Autodesk Inventor part; units mm, degrees
ref_plane "YZ Plane" through (0, 0, 0) normal (1, 0, 0) x (0, 1, 0)
ref_plane "XZ Plane" through (0, 0, 0) normal (0, 1, 0) x (-1, 0, 0)
ref_plane "XY Plane" through (0, 0, 0) normal (0, 0, 1) x (1, 0, 0)
sketch "Sketch1" plane through (0, 0, 0) normal (0, 0, 1) x (1, 0, 0)
  line L0 (-77.5, -35) -> (77.5, -35)
  line L1 (77.5, -35) -> (77.5, 35)
  line L2 (77.5, 35) -> (-77.5, 35)
  line L3 (-77.5, 35) -> (-77.5, -35)
  line L4 (-77.5, -35) -> (77.5, 35) construction
  line L5 (77.5, -35) -> (-77.5, 35) construction
  point P0 (0, 0)
  dimension "d23" = 155
  dimension "d24" = 70
extrude "Extrusion2" add sketch "Sketch1" along normal blind 5
sketch "Sketch2" plane through (0, 0, 5) normal (0, 0, 1) x (1, 0, 0)
  line L0 (-77.5, -35) -> (77.5, -35)
  line L1 (77.5, -35) -> (77.5, 35)
  line L2 (77.5, 35) -> (-77.5, 35)
  line L3 (-77.5, 35) -> (-77.5, -35)
  line L4 (-77.5, -15) -> (77.5, -15) construction
  line L5 (77.5, -35) -> (77.5, 35) construction
  circle A0 centre (0, -15) radius 7.5
  circle A1 centre (26.5, -15) radius 9.5
  line L6 (0, 35) -> (0, -35) construction
  line L7 (-77.5, -35) -> (77.5, -35) construction
  circle A2 centre (-26.5, -15) radius 9.5
  circle A3 centre (15.5455, -22) radius 3.5
  circle A4 centre (-15.5455, -8) radius 3.5
  point P0 (0, 0)
  dimension "d27" = 20
  dimension "d28" = 15
  dimension "d29" = 19
  dimension "d30" = 26.5
  dimension "d31" = 7
  dimension "d32" = 7
  dimension "d33" = 7
extrude "Extrusion3" cut sketch "Sketch2" against normal through all contours A0 | A1 | A3 | A2 | A4
sketch "Sketch3" plane through (0, 0, 5) normal (0, 0, 1) x (1, 0, 0)
  circle A0 centre (-26.5, -15) radius 9.5
  circle A1 centre (-15.5455, -8) radius 3.5
  circle A2 centre (26.5, -15) radius 9.5
  circle A3 centre (15.5455, -22) radius 3.5
  circle A4 centre (0, -15) radius 7.5
  line L0 (-77.5, -35) -> (77.5, -35)
  line L1 (77.5, -35) -> (77.5, 35)
  line L2 (77.5, 35) -> (-77.5, 35)
  line L3 (-77.5, 35) -> (-77.5, -35)
  circle A5 centre (-26.5, -15) radius 9.5
  line L4 (-20.5198, -7.6184) -> (-18.68, -6.4428)
  circle A6 centre (-15.5455, -8) radius 3.5
  line L5 (-15.5455, -8) -> (-26.5, -15) construction
  line L6 (15.5455, -22) -> (26.5, -15) construction
  circle A7 centre (15.5455, -22) radius 3.5
  line L7 (15.4493, -18.5013) -> (17.2891, -17.3257)
  line L8 (-17.2891, -12.6743) -> (-15.4493, -11.4987)
  line L9 (18.68, -23.5572) -> (20.5198, -22.3816)
  point P0 (0, 0)
  point P1 (-18.4948, -9.8846)
  point P2 (18.4948, -20.1154)
  dimension "d36" = 3
  dimension "d37" = 3
  dimension "d38" = 3
  dimension "d39" = 3
extrude "Extrusion4" cut sketch "Sketch3" against normal through all contours A0 A1 L8 | L4 A1 A0 | A2 A3 L7 | L9 A3 A2
sketch "Sketch4" plane through (0, 0, 5) normal (0, 0, 1) x (1, 0, 0)
  line L0 (-15.4493, -11.4987) -> (-17.2891, -12.6743)
  arc A0 (-20.5198, -7.6184) -> (-17.2891, -12.6743) centre (-26.5, -15) ccw
  line L1 (-20.5198, -7.6184) -> (-18.68, -6.4428)
  arc A1 (-15.4493, -11.4987) -> (-18.68, -6.4428) centre (-15.5455, -8) ccw
  line L2 (15.4493, -18.5013) -> (17.2891, -17.3257)
  arc A2 (20.5198, -22.3816) -> (17.2891, -17.3257) centre (26.5, -15) ccw
  line L3 (20.5198, -22.3816) -> (18.68, -23.5572)
  arc A3 (15.4493, -18.5013) -> (18.68, -23.5572) centre (15.5455, -22) ccw
  circle A4 centre (0, -15) radius 7.5
  line L4 (-77.5, -35) -> (77.5, -35)
  line L5 (77.5, -35) -> (77.5, 35)
  line L6 (77.5, 35) -> (-77.5, 35)
  line L7 (-77.5, 35) -> (-77.5, -35)
  line L8 (-77.5, -25) -> (77.5, -25) construction
  line L9 (-67.5, -25) -> (-47.5, -25) construction
  line L10 (-47.5, -25) -> (-47.5, 20) construction
  line L11 (-47.5, 20) -> (-67.5, 20) construction
  line L12 (-67.5, 20) -> (-67.5, -25) construction
  line L13 (77.5, 35) -> (-77.5, 35) construction
  line L14 (0, 35) -> (0, -35) construction
  circle A5 centre (-57.5, 10.5) radius 8.5
  circle A6 centre (-57.5, -15.5) radius 8.5
  line L15 (-67.5, -2.5) -> (-47.5, -2.5) construction
  line L16 (-57.5, -2.5) -> (-57.5, 10.5) construction
  line L17 (-57.5, -2.5) -> (-57.5, -15.5) construction
  circle A7 centre (57.5, 10.5) radius 8.5
  circle A8 centre (57.5, -15.5) radius 8.5
  point P0 (0, 0)
  dimension "d42" = 10
  dimension "d43" = 10
  dimension "d44" = 20
  dimension "d45" = 45
  dimension "d46" = 17
  dimension "d48" = 26
extrude "Extrusion5" cut sketch "Sketch4" against normal through all contours A5 | A6 | A7 | A8
sketch "Sketch5" plane through (0, 0, 0) normal (0, 0, -1) x (-1, 0, 0)
  circle A0 centre (-57.5, 10.5) radius 8.5
  circle A1 centre (57.5, 10.5) radius 8.5
  circle A2 centre (57.5, -15.5) radius 8.5
  circle A3 centre (-57.5, -15.5) radius 8.5
  line L0 (17.2891, -12.6743) -> (15.4493, -11.4987)
  arc A4 (18.68, -6.4428) -> (15.4493, -11.4987) centre (15.5455, -8) ccw
  line L1 (18.68, -6.4428) -> (20.5198, -7.6184)
  arc A5 (17.2891, -12.6743) -> (20.5198, -7.6184) centre (26.5, -15) ccw
  line L2 (-17.2891, -17.3257) -> (-15.4493, -18.5013)
  arc A6 (-18.68, -23.5572) -> (-15.4493, -18.5013) centre (-15.5455, -22) ccw
  line L3 (-18.68, -23.5572) -> (-20.5198, -22.3816)
  arc A7 (-17.2891, -17.3257) -> (-20.5198, -22.3816) centre (-26.5, -15) ccw
  circle A8 centre (0, -15) radius 7.5
  line L4 (77.5, -35) -> (-77.5, -35)
  line L5 (77.5, 35) -> (77.5, -35)
  line L6 (-77.5, 35) -> (77.5, 35)
  line L7 (-77.5, -35) -> (-77.5, 35)
  line L8 (-77.5, -30) -> (77.5, -30)
  line L9 (77.5, 35) -> (77.5, -35) construction
  line L10 (-77.5, -30) -> (77.5, -30)
  line L11 (77.5, -30) -> (77.5, -35)
  line L12 (77.5, -35) -> (-77.5, -35)
  line L13 (-77.5, -35) -> (-77.5, -30)
  point P0 (0, 0)
  dimension "d51" = 5
extrude "Extrusion6" add sketch "Sketch5" along normal blind 15 contours L4 L7 L8 L5
sketch "Sketch6" plane through (-77.5, -30, 0) normal (0, 1, 0) x (1, 0, 0)
  line L0 (155, 0) -> (0, 0)
  line L1 (155, 0) -> (155, 15)
  line L2 (0, 15) -> (155, 15)
  line L3 (0, 0) -> (0, 15)
  line L4 (146, 4) -> (142, 4)
  line L5 (142, 4) -> (142, 11)
  line L6 (142, 11) -> (146, 11)
  line L7 (146, 11) -> (146, 4)
  arc A0 (142, 4) -> (146, 4) centre (144, 4) ccw
  arc A1 (146, 11) -> (142, 11) centre (144, 11) ccw
  line L8 (155, 15) -> (0, 15) construction
  line L9 (77.5, 15) -> (77.5, 0) construction
  line L10 (9, 4) -> (13, 4)
  line L11 (13, 4) -> (13, 11)
  line L12 (13, 11) -> (9, 11)
  line L13 (9, 11) -> (9, 4)
  arc A2 (9, 4) -> (13, 4) centre (11, 4) ccw
  arc A3 (13, 11) -> (9, 11) centre (11, 11) ccw
  point P0 (146, 7.5)
  point P1 (155, 7.5)
  point P2 (9, 7.5)
  dimension "d54" = 4
  dimension "d55" = 7
  dimension "d56" = 9
extrude "Extrusion7" cut sketch "Sketch6" against normal through all contours A0 L4 | L4 L5 L6 L7 | L6 A1 | L13 L12 L11 L10 | L10 A2 | A3 L12
properties part number "frontPanel" material "S235"
Design review of the part built by this model. Coordinates are the model's own, in mm. A direction names the side the tool comes from. Give positions to 0.01 mm unless a question says otherwise; leave off trailing zeros. Order: outer loops, then holes, each group sorted by start corner. A loop starts at its lowest first (then second) coordinate and runs counter-clockwise, first axis right, second up. Notation, with made-up numbers: (57.25, 81.25) - (105.25, 81.25) arc R19 cw to (105.25, 104.25) - close; hole circle Ø1 at (-26, 60.25). An arc over 180 degrees is marked (long way). Use CSV: the item, a comma, the result in double quotes. Start each with the question number.
Q1. Take a section at C-C (y = 7). State the section outline as (x, z) points.
Q2. Take a section at A-A (x = 0). State the section outline as (y, z) points, and give its area (3 significant figures).
Q3. For line 1 (Y direction, x = -57.5, z = 2.45); line 2 (Y direction, x = 64, z = 0.5); line 3 (Z direction, x = -47.5, y = 2), list the stretches that pass through material, from the lowest coordinate up.
Q4. For P1, Ø12, axis at x = 24, y = 14.5, coming from the -Z side; P2, Ø2, axis at x = 48, z = -3.5, coming from the +Y side; P3, Ø24.5, axis at x = 26.5, y = -15, coming from the +Z side, all flat-tipped, find the tip position at first contact; note any pin that passes through.
Q5. Draft analysis for pull direction X (two halves, no side actions). For faces 3 (the face through (1, 35, 2)), 4 (the face through (77.5, -5.3, 0.2)), 5 (the face through (-66.5, -32.5, -2)), state which applies: pulls with the +X half, pulls with the -X half, needs draft (parallel to the pull), parting line crosses it, or undercut.
Q6. Machinability: for faces 1 (the face through (66.5, -32.5, -13)), 2 (the face through (-65.99, -15.13, 2.54)), which of the approach directions +Z, -Z, +X, -X, +Y, -Y give a long, thin tool a straight path to every point of the face, cutting with its end or side? Answer none if there is none.
Q7. Take a section at B-B (x = 52). State the section outline as (y, z) points, and give its area (3 significant figures).
Q8. Take a section at D-D (x = -44.5). State the section outline as (y, z) points.
Calculated:
1,outline,"(-77.5, 0) - (-65.25, 0) - (-65.25, 5) - (-77.5, 5) - close; (-49.75, 0) - (49.75, 0) - (49.75, 5) - (-49.75, 5) - close; (65.25, 0) - (77.5, 0) - (77.5, 5) - (65.25, 5) - close"
2,outline,"(-35, -15) - (-30, -15) - (-30, 0) - (-22.5, 0) - (-22.5, 5) - (-35, 5) - close; (-7.5, 0) - (35, 0) - (35, 5) - (-7.5, 5) - close"
2,area,"350 mm²"
3,line 1,"y = -35 to -24, -7 to 2, 19 to 35"
3,line 2,"y = -35 to -20.98, -10.02 to 5.02, 15.98 to 35"
3,line 3,"z = 0 to 5"
4,P1,"stops at z = 0"
4,P2,"stops at y = -30"
4,P3,"stops at z = 5"
5,face 3,"needs draft"
5,face 4,"pulls with the +X half"
5,face 5,"undercut"
6,face 1,"+Y, -Y"
6,face 2,"+Z, -Z"
7,outline,"(-35, -15) - (-30, -15) - (-30, 0) - (-21.98, 0) - (-21.98, 5) - (-35, 5) - close; (-9.02, 0) - (4.02, 0) - (4.02, 5) - (-9.02, 5) - close; (16.98, 0) - (35, 0) - (35, 5) - (16.98, 5) - close"
7,area,"295 mm²"
8,outline,"(-35, -15) - (-30, -15) - (-30, 0) - (35, 0) - (35, 5) - (-35, 5) - close"
